The figure shows three views and two pictorial views of one solid part (mm, origin at its lowest corner). Answer the questions. Coordinates: 2 decimals unless noted, no trailing zeros. Write each loop counter-clockwise with the first axis right and the second up, starting at its lowest first coordinate (ties: lowest second). Pieces come first, ordered by that corner, then holes. Notation, with made-up numbers: M 66,35.5 L 124,35.5 A15 cw 124,50.5 Z; hole C 54.5,-29 d8. An arc over 180 degrees is marked long. Write item = value, one per line.
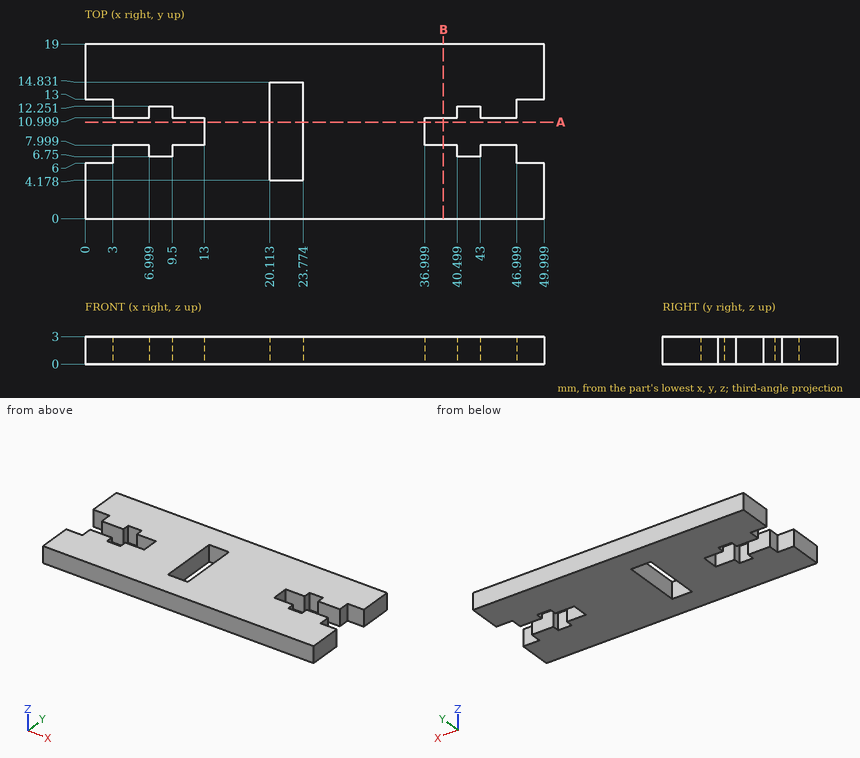
Item 1: Consider line 1 along X through (y, z) = (11.5, 2.55) (1 decimal); line 2 along X through (y, z) = (14.25, 0.2) (1 decimal); line 3 along Y through (x, z) = (45, 0.9). Determine where each line is inside the solid, lowest interval first. Write a range as from..to.
Worked answers:
line_1 = 3..7, 9.5..20.1, 23.8..40.5, 43..47
line_2 = 0..20.1, 23.8..50
line_3 = 0..8, 11..19
Item 2: Flat-ended cylindrical pins translate along their axes: pin 1 (1.4 mm diameter, centred on y = 7.5, z = 2, fed in from +X); pin 2 (0.9 mm diameter, centred on y = 9.5, z = 1.5, fed in from -X); pin 3 (1.6 mm diameter, centred on y = 7, z = 1, fed in from -X). Find the tip coordinate at first contact, or state that the pin passes through.
Worked answers:
pin_1 = 47
pin_2 = 13
pin_3 = 3
Item 3: Find section B-B (x = 39). Determine the outline of the cut face in (y, z).
Worked answers:
outline = M 0,0 L 8,0 L 8,3 L 0,3 Z; M 11,0 L 19,0 L 19,3 L 11,3 Z
Item 4: Find section A-A (y = 10.5). Determine the outline of the cut face in (x, z) (1 decimal).
Worked answers:
outline = M 13,0 L 20.1,0 L 20.1,3 L 13,3 Z; M 23.8,0 L 37,0 L 37,3 L 23.8,3 Z
